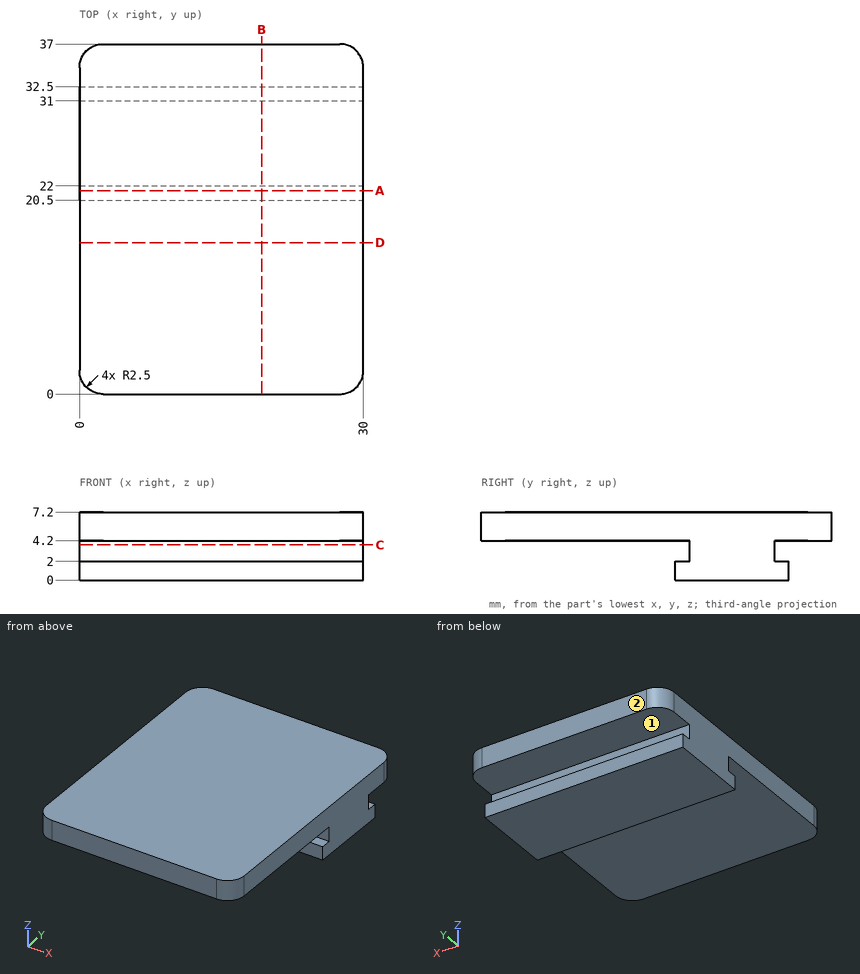
For this review, use the dimensioned drawing (mm, ordinates from the lowest corner) and the shaded views. A direction names the side the tool comes from. Round coordinates to 2 decimals unless told otherwise and drop trailing zeros. Order: outer loops, then holes, each group sorted by start corner. A loop starts at its lowest first (then second) coordinate and runs counter-clockwise, first axis right, second up. Notation, with made-up numbers: (-37.5, 4) -> (15.5, 4) arc R23 ccw to (15.5, 32) -> close; hole circle Ø4 at (-2.5, 68). An arc over 180 degrees is marked (long way). One line per item, written item: value. Start each with the question number.
Q1. Machinability: for the marked faces 1 and 2, which of the approach directions +Z, -Z, +X, -X, +Y, -Y give a long, thin tool a straight path to every point of the face, cutting with its end or side? Answer none if there is none.
Q2. Clearance check with flat-ended pins moving along their axes: pin 1 Ø10 at (x, y) = (14, 13.5) entering from -Z; pin 2 Ø1.1 at (x, z) = (18.5, 3) entering from +Y; pin 3 Ø0.6 at (x, z) = (22, 0.5) entering from +Y. State where each tip first meets the part, or that it passes through.
Q3. Take a section at A-A (y = 21.5). Write out the cut boundary in (x, z).
Q4. Take a section at D-D (y = 16). Write out the cut boundary in (x, z), and give its area (3 significant figures).
Q5. Take a section at C-C (z = 3.75). Write out the cut boundary in (x, y).
Q6. Wall thickness on line 1 (Z direction, x = 24.5, y = 17); line 2 (Y direction, x = 27, z = 4): over which ranges is each line inside the solid? List them lowest first.
Q7. Take a section at B-B (x = 19.25). Write out the cut boundary in (y, z), and give its area (3 significant figures).
Reported:
1. face 1: +X, -X, +Y
1. face 2: +Z, -Z, +X, -X, +Y
2. pin 1: stops at z = 4.2
2. pin 2: stops at y = 31
2. pin 3: stops at y = 32.5
3. outline: (0, 0) -> (30, 0) -> (30, 2) -> (0, 2) -> close; (0, 4.2) -> (30, 4.2) -> (30, 7.2) -> (0, 7.2) -> close
4. outline: (0, 4.2) -> (30, 4.2) -> (30, 7.2) -> (0, 7.2) -> close
4. area: 90.0 mm2
5. outline: (0, 22) -> (30, 22) -> (30, 31) -> (0, 31) -> close
6. line 1: z = 4.2 to 7.2
6. line 2: y = 22 to 31
7. outline: (0, 4.2) -> (22, 4.2) -> (22, 2) -> (20.5, 2) -> (20.5, 0) -> (32.5, 0) -> (32.5, 2) -> (31, 2) -> (31, 4.2) -> (37, 4.2) -> (37, 7.2) -> (0, 7.2) -> close
7. area: 155 mm2
